Study the drawing (mm; zero at the part's minimum x, y, z) and answer. A direction names the side the tool comes from. Coordinates: 2 decimals unless noted, no trailing zeros. Order: outer loops, then holes, each group sorted by start corner. A loop starts at its lowest first (then second) coordinate and runs counter-clockwise, first axis right, second up. Notation, with made-up numbers: (87.25, 88) -> (93.25, 88) arc R27 ccw to (93.25, 118) -> close; hole circle Ø5 at (6.5, 38). An arc over 180 degrees is marked (long way). Put each result on its own line as item: value. Start each with the question number.
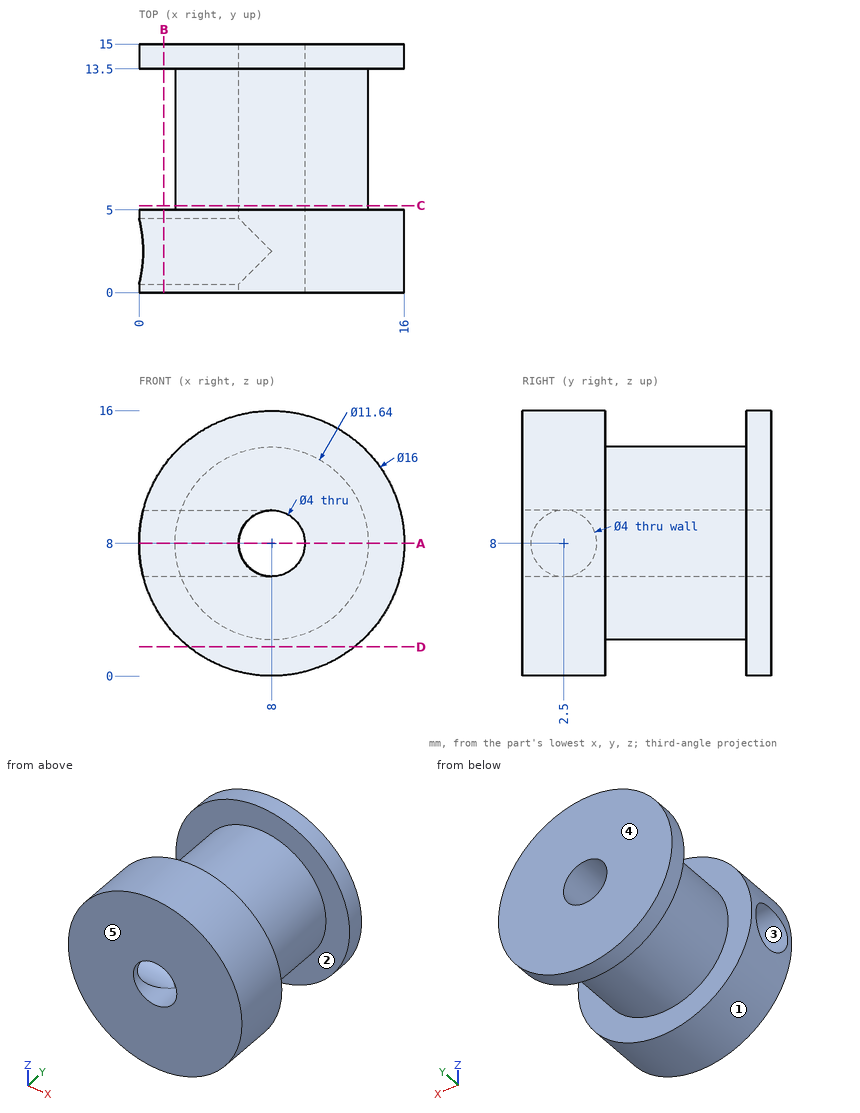
(1) A tool of negligible diameter and unlimited length cuts with its end or side. For the marked faces 1 and 2, from which of +Z, -Z, +X, -X, +Y, -Y can it reach the whole face along a straight path? Write none if from no direction.
(2) The part is cut by section B-B on x = 1.5. Determine the outline of the cut face in (y, z).
(3) Find the intervals of material crossed by L1, parallel to Z at x = 8, y = 10; L2, parallel to Y at x = 14.5, z = 5.75; L3, parallel to Z at x = 8, y = 4, in increasing order.
(4) Each of these flat-tipped pins is pushed along its axis until it touches: P1, Ø3.5, axis at y = 2.5, z = 8, coming from the -X side; P2, Ø2, axis at y = 8.5, z = 2, coming from the +X side; P3, Ø1, axis at y = 13.5, z = 5.5, coming from the -X side. Where does it stop, or does it pass through?
(5) For a pull along Y with two mould halves and no side action, classify the marked faces 3, 4 and 5 as released by +Y, released by -Y, zero draft, split by the parting line, or undercut.
(6) The part is cut by section C-C on y = 5.25. Determine the outline of the cut face in (x, z), plus the area to 3 significant figures.
(7) The part is cut by section A-A on z = 8. Determine the outline of the cut face in (x, y).
(8) The part is cut by section D-D on z = 1.75. Determine the outline of the cut face in (x, y).
Worked out:
1. face 1: +Y, -Y
1. face 2: none
2. outline: (0, 3.34) -> (5, 3.34) -> (5, 12.66) -> (0, 12.66) -> close; (13.5, 3.34) -> (15, 3.34) -> (15, 12.66) -> (13.5, 12.66) -> close; hole circle Ø4 at (2.5, 8)
3. L1: 2.18 to 6, 10 to 13.82
3. L2: 0 to 5, 13.5 to 15
3. L3: 0 to 6, 10 to 16
4. P1: x = 8.97
4. P2: x = 10.98
4. P3: x = 0.25
5. face 3: undercut
5. face 4: released by +Y
5. face 5: released by -Y
6. outline: circle Ø11.64 at (8, 8); hole circle Ø4 at (8, 8)
6. area: 93.8 mm2
7. outline: (0, 0) -> (6, 0) -> (6, 0.5) -> (0, 0.5) -> close; (0, 4.5) -> (6, 4.5) -> (6, 15) -> (0, 15) -> (0, 13.5) -> (2.18, 13.5) -> (2.18, 5) -> (0, 5) -> close; (10, 0) -> (16, 0) -> (16, 5) -> (13.82, 5) -> (13.82, 13.5) -> (16, 13.5) -> (16, 15) -> (10, 15) -> close
8. outline: (3.01, 0) -> (12.99, 0) -> (12.99, 5) -> (3.01, 5) -> close; (3.01, 13.5) -> (12.99, 13.5) -> (12.99, 15) -> (3.01, 15) -> close
